Work out the finished part from the listing and answer in its coordinate system (mm). A direction names the side the tool comes from. Give positions to 0.01 mm unless a question says otherwise; leave off trailing zeros. Order: outer loops, then holes, each group sorted by start corner. A loop starts at its lowest first (then second) coordinate and runs counter-clockwise, first axis right, second up. Notation, with made-up numbers: (-19.5, 9.25) - (-8.5, 9.25) arc R25 ccw to (-8.5, 32.25) - close; hole circle Ø4 at (25.25, 12). An arc over 180 degrees is marked (long way). Put each result on its own line as item: value.
```python
from build123d import *

# Parameters (mm, degrees)
SKETCH_1_R      = 3.5
SKETCH_1_R_2    = 1.8
EXTRUDE_1_DEPTH = 3
SKETCH_1_3_R    = 1.8
EXTRUDE_2_DEPTH = 26
CHAMFER_1_SIZE  = 1


with BuildPart() as part:
    # Sketch 1 → Extrude 1 (new body)
    with BuildSketch(Plane(origin=(0, 0, 0), x_dir=(1, 0, 0), z_dir=(0, 1, 0))):
        with Locations(Location((0, 0, 0), (0, 0, 270))):
            Circle(SKETCH_1_R)
        Circle(SKETCH_1_R_2, mode=Mode.SUBTRACT)
        Circle(SKETCH_1_R_2)
    extrude(amount=-EXTRUDE_1_DEPTH)

    # Sketch 1_3 → Extrude 2 (add)
    with BuildSketch(Plane(origin=(0, 0, 0), x_dir=(1, 0, 0), z_dir=(0, 1, 0))):
        with Locations(Location((0, 0, 0), (0, 0, 90))):
            Circle(SKETCH_1_3_R)
    extrude(amount=EXTRUDE_2_DEPTH)

    # Chamfer 1
    chamfer_1_edges = [part.edges().sort_by_distance(p)[0] for p in [
        (0, 26, 1.8),
    ]]
    chamfer(chamfer_1_edges, length=CHAMFER_1_SIZE)


solid = part.part
```
(1) Section D-D, the plane x = -2.25 is taken. Write down the section's boundary in (y, z).
Geometry check:
outline: (-3, -2.68) - (0, -2.68) - (0, 2.68) - (-3, 2.68) - close
(2) Section C-C, the plane y = 21.25 is taken. Write down the section's boundary in (x, z), then the cut area to 3 significant figures.
Geometry check:
outline: circle Ø3.6 at (0, 0)
area: 10.2 mm²
(3) Section A-A, the plane x = 0 is taken. Write down the section's boundary in (y, z).
Geometry check:
outline: (-3, -3.5) - (0, -3.5) - (0, -1.8) - (25, -1.8) - (26, -0.8) - (26, 0.8) - (25, 1.8) - (0, 1.8) - (0, 3.5) - (-3, 3.5) - close
(4) Straight lines are drawn through the part: line 1 (Y direction, x = 1, z = 2.75); line 2 (X direction, y = 14, z = 0); line 3 (Z direction, x = 1.25, y = 23.75). For each, find the intervals that lie inside material, in ascending order.
Geometry check:
line 1: y = -3 to 0
line 2: x = -1.8 to 1.8
line 3: z = -1.3 to 1.3
(5) A tool of negligible diameter and unlimited length cuts with its end or side. For faces 1 (the face through (0.689, 12.325, -1.663)), 2 (the face through (0, 26, 0)), from which of +Z, -Z, +X, -X, +Y, -Y can it reach the whole face along a straight path? Write none if from no direction.
Geometry check:
face 1: +Y
face 2: +Z, -Z, +X, -X, +Y
(6) Given pin 1 (2 mm diameter, centred on x = -2, y = 18.5, fed in from +Z); pin 2 (4 mm diameter, centred on x = -1, y = 13, fed in from +Z); pin 3 (4 mm diameter, centred on x = -0.5, z = 2, fed in from +Y); pin 4 (2 mm diameter, centred on y = 19, z = 0, fed in from -X), each flat-ended and moving along its own axis, determine where each tip first touches the part or whether it passes through.
Geometry check:
pin 1: stops at z = 1.5
pin 2: stops at z = 1.8
pin 3: stops at y = 26
pin 4: stops at x = -1.8
(7) Section B-B, the plane z = 0 is taken. Write down the section's boundary in (x, y).
Geometry check:
outline: (-3.5, -3) - (3.5, -3) - (3.5, 0) - (1.8, 0) - (1.8, 25) - (0.8, 26) - (-0.8, 26) - (-1.8, 25) - (-1.8, 0) - (-3.5, 0) - close
